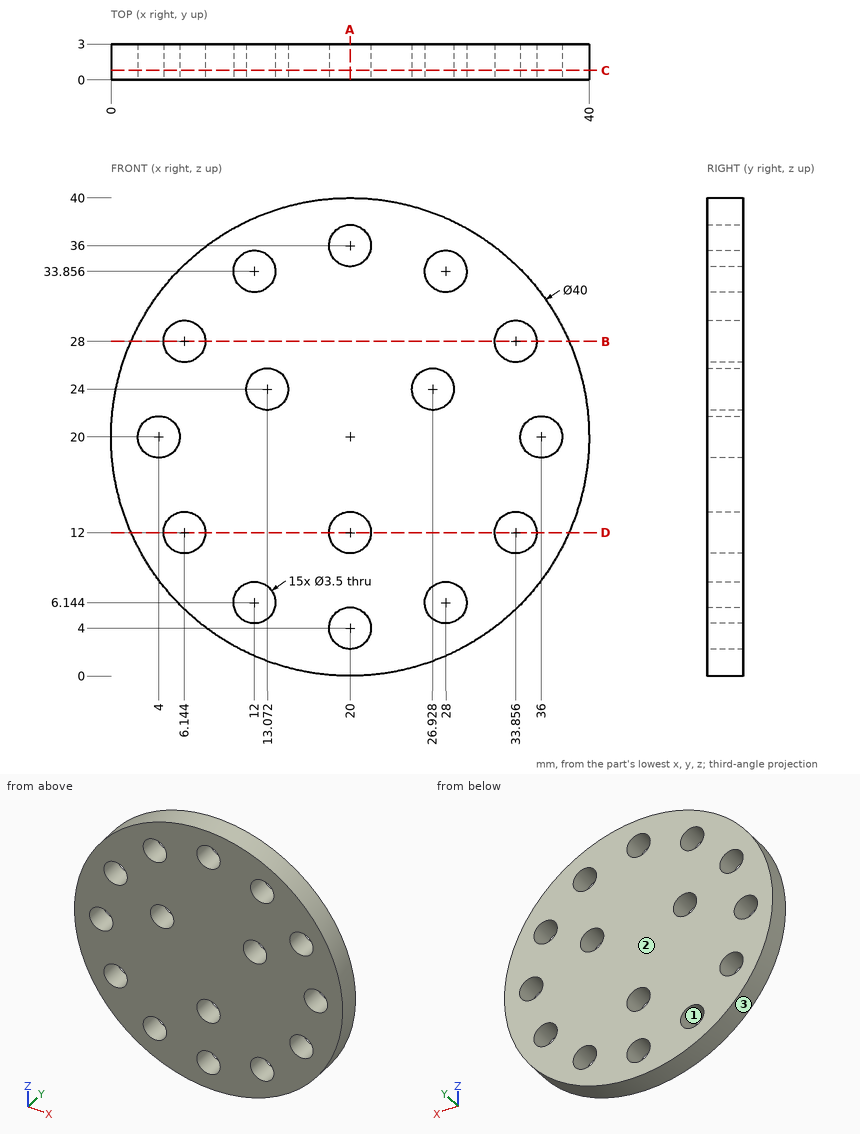
Geometry check sheet. Reference: drawing and pictorial views, mm from the part's lowest x, y, z. Give positions to 0.01 mm unless a question says otherwise; leave off trailing zeros. Order: outer loops, then holes, each group sorted by start corner. A loop starts at its lowest first (then second) coordinate and runs counter-clockwise, first axis right, second up. Notation, with made-up numbers: M 53.5,39.5 L 100.5,39.5 A23 ccw 100.5,78.5 Z; hole C 21.5,-29 d1. An arc over 180 degrees is marked long. Answer in a Markdown table with one row per item.
1) Release check for a two-part mould opening along X. For the marked faces 1, 2 and 3 record: +X half, -X half, draft (parallel to the pull), parting line (faces both ways), or undercut.
Filled sheet:
| item | result |
|---|---|
| face 1 | undercut |
| face 2 | draft |
| face 3 | parting line |
2) Thickness scan on L1, parallel to X at y = 1.6, z = 24 (1 decimal); L2, parallel to X at y = 2.4, z = 35 (1 decimal); L3, parallel to X at y = 0.35, z = 34 (1 decimal). Record the ranges inside material, lowest first. Write a range as [from, to].
Filled sheet:
| item | result |
|---|---|
| L1 | x = [0.4, 11.3], [14.8, 25.2], [28.7, 39.6] |
| L2 | x = [6.8, 10.7], [13.3, 18.6], [21.4, 26.7], [29.3, 33.2] |
| L3 | x = [5.7, 10.3], [13.7, 26.3], [29.7, 34.3] |
3) Cross-section at C-C, the plane y = 0.8. Count the separate pieces of the cut face and the enclosed holes in it, plus the area to 3 significant figures.
Filled sheet:
| item | result |
|---|---|
| separate pieces | 1 |
| enclosed holes | 15 |
| area | 1,110 mm2 |
4) Gauge pin test, flat ends, axial feed: P1, Ø2, axis at x = 6.14, z = 12, coming from the -Y side; P2, Ø1, axis at y = 0.5, z = 29, coming from the -X side. Record the tip position at first contact, or that the pin passes through.
Filled sheet:
| item | result |
|---|---|
| P1 | passes through |
| P2 | stops at x = 1.9 |
5) Cross-section at B-B, the plane z = 28. Enter the section's corners in (x, y).
Filled sheet:
| item | result |
|---|---|
| outline | M 1.67,0 L 4.39,0 L 4.39,3 L 1.67,3 Z; M 7.89,0 L 32.11,0 L 32.11,3 L 7.89,3 Z; M 35.61,0 L 38.33,0 L 38.33,3 L 35.61,3 Z |
6) Cross-section at D-D, the plane z = 12. Enter the section's corners in (x, y).
Filled sheet:
| item | result |
|---|---|
| outline | M 1.67,0 L 4.39,0 L 4.39,3 L 1.67,3 Z; M 7.89,0 L 18.25,0 L 18.25,3 L 7.89,3 Z; M 21.75,0 L 32.11,0 L 32.11,3 L 21.75,3 Z; M 35.61,0 L 38.33,0 L 38.33,3 L 35.61,3 Z |
7) Cross-section at A-A, the plane x = 20. Enter the section's corners in (y, z).
Filled sheet:
| item | result |
|---|---|
| outline | M 0,0 L 3,0 L 3,2.25 L 0,2.25 Z; M 0,5.75 L 3,5.75 L 3,10.25 L 0,10.25 Z; M 0,13.75 L 3,13.75 L 3,34.25 L 0,34.25 Z; M 0,37.75 L 3,37.75 L 3,40 L 0,40 Z |
